from build123d import *

# Parameters (mm, degrees)
F1_DEPTH = 27.8131016
F2_R     = 3.69316
F3_R     = 1.98374
F5_DEPTH = 32.78124
F6_R     = 1.35255
F7_DEPTH = 1.70942
F8_R     = 4.41325


with BuildPart() as f1:
    # F0 (on Top) → F1 (new body)
    with BuildSketch(Plane.XY):
        Polygon((0, 16.8191942), (0, 0), (-29.3624, 0), (-29.3624, 16.8191942), (-31.07182, 16.8191942), (-31.07182, -1.70942), (1.70942, -1.70942), (1.70942, 16.8191942), align=None)
    extrude(amount=F1_DEPTH)

    # F2
    f2_edges = [f1.edges().sort_by_distance(p)[0] for p in [
        (1.70942, -1.70942, 13.906551),
        (-31.07182, -1.70942, 13.906551),
    ]]
    fillet(f2_edges, radius=F2_R)

    # F3
    f3_edges = [f1.edges().sort_by_distance(p)[0] for p in [
        (0, 0, 13.906551),
        (-29.3624, 0, 13.906551),
    ]]
    fillet(f3_edges, radius=F3_R)

    # F4 (on face) → F5 (cut, through all)
    with BuildSketch(Plane.YZ.offset(1.70942)):
        with BuildLine():
            Line((10.7121942, 24.5224534606), (10.7121942, 22.2772497394))
            ThreePointArc((10.7121942, 22.2772497394), (14.4379442, 23.3998516), (10.7121942, 24.5224534606))
        make_face()
        with BuildLine():
            Line((10.7121942, 5.5358518606), (10.7121942, 3.2906481394))
            ThreePointArc((10.7121942, 3.2906481394), (14.4379442, 4.41325), (10.7121942, 5.5358518606))
        make_face()
    extrude(amount=-F5_DEPTH, mode=Mode.SUBTRACT)

    # F6 (on face) → F7 (cut, through all)
    with BuildSketch(Plane.XZ.offset(1.70942)):
        with BuildLine():
            ThreePointArc((-6.5960560047, 27.4691345745), (-5.8976903725, 27.7259126932), (-5.15874, 27.8131016))
            Line((-5.15874, 27.8131016), (-24.20366, 27.8131016))
            ThreePointArc((-24.20366, 27.8131016), (-23.4647096275, 27.7259126932), (-22.7663439953, 27.4691345745))
            ThreePointArc((-22.7663439953, 27.4691345745), (-14.6812, 25.5342622696), (-6.5960560047, 27.4691345745))
        make_face()
        with Locations((-24.20366, 24.6381016)):
            Circle(F6_R)
        with Locations((-5.15874, 24.6381016)):
            Circle(F6_R)
        with Locations((-24.20366, 3.175)):
            Circle(F6_R)
        with Locations((-5.15874, 3.175)):
            Circle(F6_R)
    extrude(amount=-F7_DEPTH, mode=Mode.SUBTRACT)

    # F8
    f8_edges = [f1.edges().sort_by_distance(p)[0] for p in [
        (0.85471, 16.819194, 27.813102),
        (-30.21711, 16.819194, 27.813102),
        (0.85471, 16.819194, 0),
        (-30.21711, 16.819194, 0),
    ]]
    fillet(f8_edges, radius=F8_R)


solid = f1.part
Read the model definition and answer for the solid it produces. Units are mm, in the model's axes. A direction names the side the tool comes from. Round coordinates to 2 decimals unless told otherwise and drop trailing zeros. Order: outer loops, then holes, each group sorted by start corner. A loop starts at its lowest first (then second) coordinate and runs counter-clockwise, first axis right, second up.
1) The part is cut by section A-A on y = 4.25. Write down the section's boundary in (x, z), plus the area to 3 significant figures.
2) Straight lines are drawn through the part: L1, parallel to X at y = 3.75, z = 13.75; L2, parallel to Y at x = -4, z = 11.5; L3, parallel to X at y = 1, z = 20. For each, find the intervals that lie inside material, in ascending order.
3) The part is cut by section C-C on x = -23.5. Write down the section's boundary in (y, z), plus the area to 3 significant figures.
4) Flat-ended cylindrical pins translate along their axes: pin 1 (0.5 mm diameter, centred on x = 0.5, z = 24, fed in from +Y); pin 2 (8 mm diameter, centred on x = -11, y = 1, fed in from +Z). Find the tip coordinate at first contact, or state that the pin passes through.
5) The mould has two halves that part along Y. Classify faces 1 (the face through (-30.205, 14.437, 4.341)), 2 (the face through (0, 10, 14)), 3 (the face through (-30, 10.712, 23)), 4 (the face through (-0.597, 0.566, 14.101)): released by +Y, released by -Y, zero draft, split by the parting line, or undercut.
6) The part is cut by section D-D on x = -27. Write down the section's boundary in (y, z), plus the area to 3 significant figures.
7) For faces 5 (the face through (1, 10.712, 23)), 6 (the face through (-15, 0, 14)), 7 (the face through (-30, 4, 27.813)), 8 (the face through (-23.475, -0.867, 27.728)), 9 (the face through (-31.072, 10, 14)), determine the directions among +Z, -Z, +X, -X, +Y, -Y from which every point of the face is accessible in a straight line to the end or side of a thin tool.
8) The part is cut by section B-B on z = 18.75. Write down the section's boundary in (x, y).
Resolved:
1. outline: (-31.07, 0) - (-29.36, 0) - (-29.36, 27.81) - (-31.07, 27.81) - close; (0, 0) - (1.71, 0) - (1.71, 27.81) - (0, 27.81) - close
1. area: 95.1 mm2
2. L1: x = -31.07 to -29.36, 0 to 1.71
2. L2: y = -1.71 to 0
2. L3: x = -30.94 to -29.1, -0.26 to 1.58
3. outline: (-1.71, 0) - (0, 0) - (0, 2.02) - (-1.71, 2.02) - close; (-1.71, 4.33) - (0, 4.33) - (0, 23.48) - (-1.71, 23.48) - close; (-1.71, 25.79) - (0, 25.79) - (0, 27.73) - (-1.71, 27.73) - close
3. area: 39.5 mm2
4. pin 1: stops at y = 16.81
4. pin 2: stops at z = 27.21
5. face 1: undercut
5. face 2: zero draft
5. face 3: undercut
5. face 4: released by +Y
6. outline: (-1.71, 0) - (0, 0) - (0, 27.81) - (-1.71, 27.81) - close
6. area: 47.5 mm2
7. face 5: +X, -X
7. face 6: +Z, -Z, +Y
7. face 7: +Z, +X, -X, +Y, -Y
7. face 8: +Z, +Y, -Y
7. face 9: +Z, -Z, -X, +Y, -Y
8. outline: (-31.07, 1.98) arc R3.69 ccw to (-27.38, -1.71) - (-1.98, -1.71) arc R3.69 ccw to (1.71, 1.98) - (1.71, 16.82) - (0, 16.82) - (0, 1.98) arc R1.98 cw to (-1.98, 0) - (-27.38, 0) arc R1.98 cw to (-29.36, 1.98) - (-29.36, 16.82) - (-31.07, 16.82) - close
